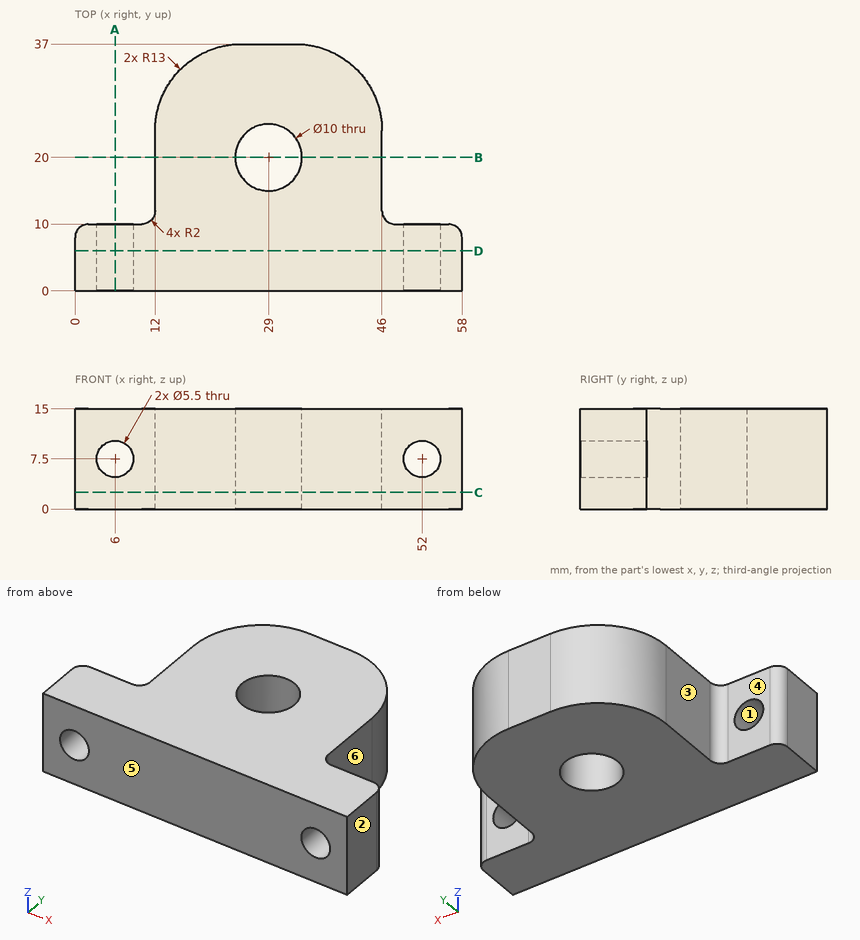
Here's the drawing with two shaded views (mm, measured from the low corner). I have some questions. A direction names the side the tool comes from. Give positions to 0.01 mm unless a question says otherwise; leave off trailing zeros. Write each loop counter-clockwise with the first axis right and the second up, starting at its lowest first coordinate (ties: lowest second). Pieces come first, ordered by that corner, then holes. Notation, with made-up numbers: (34, 63) - (44, 63) arc R16 cw to (44, 72) - close; hole circle Ø5 at (37, -4). An arc over 180 degrees is marked (long way). One line per item, written item: value. Start each with the question number.
Item 1: Imagine slicing it at A-A, the plane x = 6. List the corners of the cut face in (y, z) for me.
Item 2: If we mould it in two halves opening along X, with no side actions, what happens to the marked faces 1, 2 and 3? For each: +X half, -X half, draft (parallel to the pull), parting line (faces both ways), or undercut.
Item 3: Imagine slicing it at B-B, the plane y = 20. List the corners of the cut face in (x, z) for me, and give its area (3 significant figures).
Item 4: Which directions (+Z, -Z, +X, -X, +Y, -Y) give clear straight access to the entire face, cutting with the end or side of a thin tool? Please do the marked faces 4, 5 and 6.
Item 5: Please list where these lines run through material, in increasing order: line 1 (X direction, y = 6, z = 7.5); line 2 (Z direction, x = 52, y = 5); line 3 (X direction, y = 6, z = 9). Write a range as from..to.
Item 6: Imagine slicing it at C-C, the plane z = 2.5. List the corners of the cut face in (x, y) for me, and give its area (3 significant figures).
Item 7: I'm going to push flat-ended pins straight in: pin 1 (6.5 mm diameter, centred on x = 53, z = 5.5, fed in from +Y); pin 2 (1 mm diameter, centred on x = 33, y = 21, fed in from +Z); pin 3 (1 mm diameter, centred on x = 41.5, z = 2, fed in from +Y); pin 4 (6 mm diameter, centred on y = 20.5, z = 4.5, fed in from -X). Where does each tip first touch, or does it pass through?
Item 8: Imagine slicing it at D-D, the plane y = 6. List the corners of the cut face in (x, z) for me.
Geometry says:
1. outline: (0, 0) - (10, 0) - (10, 4.75) - (0, 4.75) - close; (0, 10.25) - (10, 10.25) - (10, 15) - (0, 15) - close
2. face 1: undercut
2. face 2: +X half
2. face 3: -X half
3. outline: (12, 0) - (24, 0) - (24, 15) - (12, 15) - close; (34, 0) - (46, 0) - (46, 15) - (34, 15) - close
3. area: 360 mm^2
4. face 4: +Z, -Z, -X, +Y
4. face 5: +Z, -Z, +X, -X, -Y
4. face 6: +Z, -Z, +X, +Y
5. line 1: 0..3.25, 8.75..49.25, 54.75..58
5. line 2: 0..4.75, 10.25..15
5. line 3: 0..3.7, 8.3..49.7, 54.3..58
6. outline: (0, 0) - (58, 0) - (58, 8) arc R2 ccw to (56, 10) - (48, 10) arc R2 cw to (46, 12) - (46, 24) arc R13 ccw to (33, 37) - (25, 37) arc R13 ccw to (12, 24) - (12, 12) arc R2 cw to (10, 10) - (2, 10) arc R2 ccw to (0, 8) - close; hole circle Ø10 at (29, 20)
6. area: 1,350 mm^2
7. pin 1: y = 10
7. pin 2: through
7. pin 3: y = 34.25
7. pin 4: x = 12
8. outline: (0, 0) - (58, 0) - (58, 15) - (0, 15) - close; hole circle Ø5.5 at (6, 7.5); hole circle Ø5.5 at (52, 7.5)
